from build123d import *

# Parameters (mm, degrees)
ESQUISSE1_R             = 2.5
ESQUISSE1_W             = 40
ESQUISSE1_H             = 8
BOSS_EXTRU_1_DEPTH      = 6
ESQUISSE2_R             = 2.5
BOSS_EXTRU_2_DEPTH      = 8
CONG_2_R                = 2
ENL_V_MAT_EXTRU_1_DEPTH = 4
ENL_V_START             = -10
ENL_V_MAT_EXTRU_4_DEPTH = 10


with BuildPart() as part:
    # Esquisse1 → Boss.-Extru.1 (new body)
    with BuildSketch(Plane.XY):
        with BuildLine():
            Line((90, -15), (-90, -15))
            ThreePointArc((-90, -15), (-105, 0), (-90, 15))
            Line((-90, 15), (90, 15))
            ThreePointArc((90, 15), (105, 0), (90, -15))
        make_face()
        with Locations((99, 0)):
            Circle(ESQUISSE1_R, mode=Mode.SUBTRACT)
        with Locations(Location((-90, 0, 0), (0, 0, 180))):
            Circle(ESQUISSE1_R, mode=Mode.SUBTRACT)
        with BuildLine():
            Line((0, -2.5), (-75, -2.5))
            ThreePointArc((-75, -2.5), (-77.5, 0), (-75, 2.5))
            Line((-75, 2.5), (0, 2.5))
            Line((0, 2.5), (15, 2.5))
            ThreePointArc((15, 2.5), (17.5, 0), (15, -2.5))
            Line((15, -2.5), (0, -2.5))
        make_face(mode=Mode.SUBTRACT)
        with Locations((60, 0)):
            Rectangle(ESQUISSE1_W, ESQUISSE1_H, mode=Mode.SUBTRACT)
    extrude(amount=BOSS_EXTRU_1_DEPTH)

    # Esquisse2 → Boss.-Extru.2 (add)
    with BuildSketch(Plane(origin=(40, 0, 0), x_dir=(0, 0, -1), z_dir=(1, 0, 0))):
        Polygon((-16, 5), (-16, -5), (-6, -15), (-6, -5), (-6, 5), (-6, 15), align=None)
        with Locations((-11, 0)):
            Circle(ESQUISSE2_R, mode=Mode.SUBTRACT)
    extrude(amount=-BOSS_EXTRU_2_DEPTH)

    # Congé2
    cong_2_edges = [part.edges().sort_by_distance(p)[0] for p in [
        (40, 9.5, 6),
        (40, -9.5, 6),
    ]]
    fillet(cong_2_edges, radius=CONG_2_R)

    # Esquisse3 → Enlèv. mat.-Extru.1 (cut)
    with BuildSketch(Plane.ZY.offset(-32)):
        Polygon((11, 4), (14.464101615, 2), (14.464101615, -2), (11, -4), (7.535898385, -2), (7.535898385, 2), align=None)
    extrude(amount=-ENL_V_MAT_EXTRU_1_DEPTH, mode=Mode.SUBTRACT)

    # Esquisse4 → Enlèv. mat.-Extru.4 (cut)
    with BuildSketch(Plane.XY.offset(6).offset(ENL_V_START)):
        with BuildLine():
            ThreePointArc((-105, 0), (-104.771638598, -1.148050297), (-104.121320344, -2.121320344))
            Line((-104.121320344, -2.121320344), (-99.878679656, 2.121320344))
            ThreePointArc((-99.878679656, 2.121320344), (-103.148050297, 2.771638598), (-105, 0))
        make_face()
        with BuildLine():
            Line((-99.878679656, 2.121320344), (-104.121320344, -2.121320344))
            ThreePointArc((-104.121320344, -2.121320344), (-100.851949703, -2.771638598), (-99, 0))
            ThreePointArc((-99, 0), (-99.228361402, 1.148050297), (-99.878679656, 2.121320344))
        make_face()
        with BuildLine():
            ThreePointArc((-105, 0), (-103.148050297, 2.771638598), (-99.878679656, 2.121320344))
            Line((-99.878679656, 2.121320344), (-103.750652313, 5.993293))
            ThreePointArc((-103.750652313, 5.993293), (-104.68434174, 3.061063158), (-105, 0))
        make_face()
        with BuildLine():
            Line((-104.94364809, -1.298992597), (-104.121320344, -2.121320344))
            ThreePointArc((-104.121320344, -2.121320344), (-104.771638598, -1.148050297), (-105, 0))
            ThreePointArc((-105, 0), (-104.985905401, -0.650107165), (-104.94364809, -1.298992597))
        make_face()
        with BuildLine():
            ThreePointArc((-105, 0), (-104.771638598, -1.148050297), (-104.121320344, -2.121320344))
            Line((-104.121320344, -2.121320344), (-99.878679656, 2.121320344))
            ThreePointArc((-99.878679656, 2.121320344), (-103.148050297, 2.771638598), (-105, 0))
        make_face()
        with BuildLine():
            Line((-99.878679656, 2.121320344), (-104.121320344, -2.121320344))
            ThreePointArc((-104.121320344, -2.121320344), (-100.851949703, -2.771638598), (-99, 0))
            ThreePointArc((-99, 0), (-99.228361402, 1.148050297), (-99.878679656, 2.121320344))
        make_face()
    extrude(amount=ENL_V_MAT_EXTRU_4_DEPTH, mode=Mode.SUBTRACT)


solid = part.part
Model file for the job. Use its own axes, mm. A direction names the side the tool comes from. Round coordinates to 2 decimals unless told otherwise and drop trailing zeros. Order: outer loops, then holes, each group sorted by start corner. A loop starts at its lowest first (then second) coordinate and runs counter-clockwise, first axis right, second up.
(1) Band-saw the part on A-A (z = 4.25). List the corners of the cut face in (x, y).
(2) Band-saw the part on B-B (x = -12). List the corners of the cut face in (y, z).
(3) Band-saw the part on D-D (x = 49). List the corners of the cut face in (y, z).
(4) Drill centre lines: line 1 (Y direction, x = 42, z = 5.5); line 2 (Y direction, x = -90, z = 4); line 3 (Z direction, x = 31, y = 0). Where is each one in solid material? Low to high.
(5) Pin check, flat tips, straight feed: pin 1 (6 mm diameter, centred on y = 0, z = 11, fed in from -X); pin 2 (3 mm diameter, centred on y = -10, z = 3, fed in from -X); pin 3 (15 mm diameter, centred on x = 73, y = 0, fed in from +Z). Stop position of each tip, or through.
(6) 3-axis set-ups, long thin cutter, end or side, ignore diameter. For faces 4 (the face through (-101.79, 4.03, 2.96)), 5 (the face through (17.5, 0.1, 3)), 6 (the face through (38, 0.1, 13.5)), 7 (the face through (32, -3.1, 8.8)), 8 (the face through (33.972, 2.986, 9.244)): which of +Z, -Z, +X, -X, +Y, -Y reach the whole face in a straight line?
(7) Pull direction X, two halves, no side cores. Call faces 1 (the face through (-87.5, -0.1, 3)), 2 (the face through (34, 0, 7.536)), 3 (the face through (-98.32, 12.48, 2.96)): released by +X, released by -X, zero draft, split by the parting line, or undercut.
(8) Band-saw the part on C-C (y = 10). List the corners of the cut face in (x, z).
Verdict:
1. outline: (-104.94, -1.3) arc R15 ccw to (-90, -15) - (90, -15) arc R15 ccw to (90, 15) - (-90, 15) arc R15 ccw to (-103.75, 5.99) - (-99.88, 2.12) arc R3 cw to (-104.12, -2.12) - close; hole circle Ø5 at (-90, 0); hole (-75, -2.5) - (15, -2.5) arc R2.5 ccw to (15, 2.5) - (-75, 2.5) arc R2.5 ccw to start; hole (40, -4) - (80, -4) - (80, 4) - (40, 4) - close; hole circle Ø5 at (99, 0)
2. outline: (-15, 0) - (-2.5, 0) - (-2.5, 6) - (-15, 6) - close; (2.5, 0) - (15, 0) - (15, 6) - (2.5, 6) - close
3. outline: (-15, 0) - (-4, 0) - (-4, 6) - (-15, 6) - close; (4, 0) - (15, 0) - (15, 6) - (4, 6) - close
4. line 1: y = -15 to -4, 4 to 15
4. line 2: y = -15 to -2.5, 2.5 to 15
4. line 3: z = 0 to 6
5. pin 1: stops at x = 36
5. pin 2: stops at x = -102.36
5. pin 3: stops at z = 6
6. face 4: +Z, -Z, -X
6. face 5: +Z, -Z
6. face 6: +X, -X
6. face 7: +Z, -X, +Y, -Y
6. face 8: -X
7. face 1: undercut
7. face 2: zero draft
7. face 3: released by -X
8. outline: (-101.18, 0) - (101.18, 0) - (101.18, 6) - (42, 6) arc R2 cw to (40, 8) - (40, 11) - (32, 11) - (32, 6) - (-101.18, 6) - close
